The drawing under review shows one solid part. Ordinate dimensions are in mm from its lowest x, y, z. A direction names the side the tool comes from. Give positions to 0.01 mm unless a question says otherwise; leave off trailing zeros. Order: outer loops, then holes, each group sorted by start corner. A loop starts at its lowest first (then second) coordinate and runs counter-clockwise, first axis right, second up. Notation, with made-up numbers: (-7.5, -21.5) - (13.5, -21.5) arc R14 cw to (13.5, 0.5) - close; hole circle Ø8 at (54, -31). An arc over 180 degrees is marked (long way). Answer as a JSON object with one key per item and string values. Group by question number.
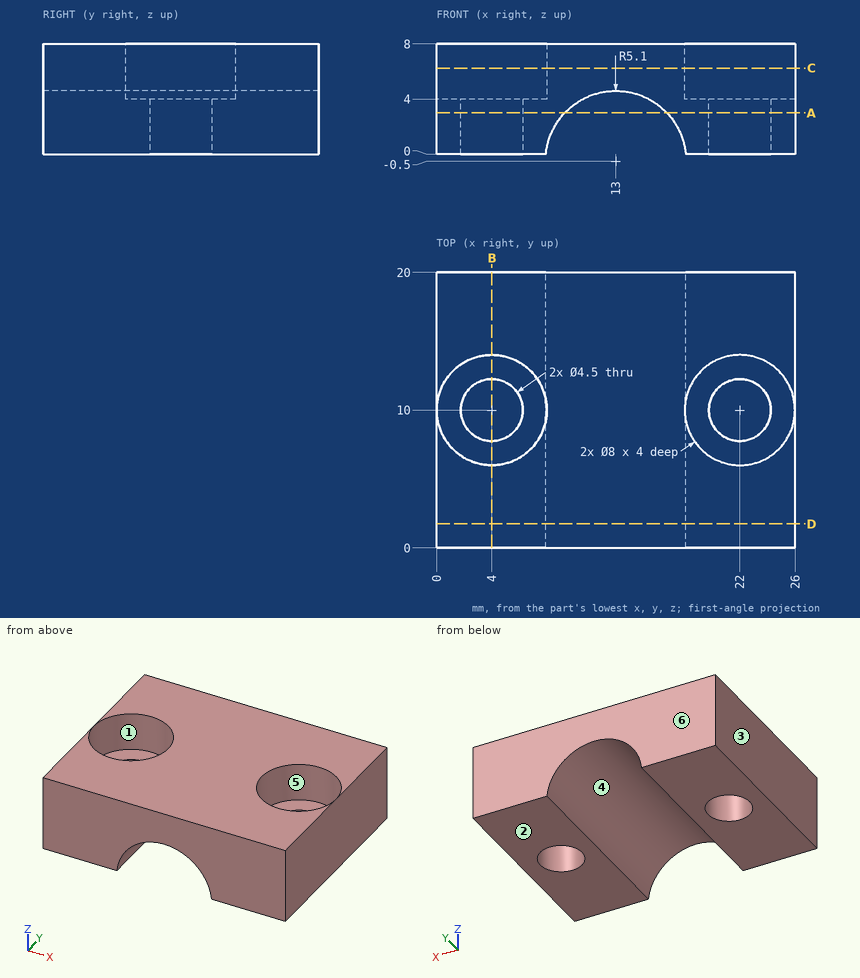
1) For line 1 (Y direction, x = 4, z = 2.1); line 2 (Y direction, x = 22, z = 6.75); line 3 (X direction, y = 10, z = 1.9), list the stretches that pass through material, from the lowest coordinate up.
2) Consider section C-C (z = 6.25). Give the boundary of the cut face in (x, y).
3) Consider section B-B (x = 4). Give the boundary of the cut face in (y, z).
4) Consider section A-A (z = 3). Give the boundary of the cut face in (x, y), plus the area to 3 significant figures.
5) For the marked faces 5 and 6, list the 3-axis set-ups (+Z, -Z, +X, -X, +Y, -Y) from which the entire face can be reached by the end or side of a thin tool; tool diameter is ignored.
6) For pin 1 (2.5 mm diameter, centred on x = 20.5, y = 11, fed in from +Z); pin 2 (9 mm diameter, centred on x = 4, y = 11.5, fed in from +Z); pin 3 (2.5 mm diameter, centred on x = 4, y = 10, fed in from +Z), all flat-tipped, find the tip position at first contact; note any pin that passes through.
7) Consider section D-D (y = 1.75). Give the boundary of the cut face in (x, z), plus the area to 3 significant figures.
8) Mouldability with a two-part tool opening along X and no side actions: class the marked faces 1, 2, 3 and 4 as released by +X, released by -X, zero draft, split by the parting line, or undercut.
Result set:
{
 "1": {"line 1": "y = 0 to 7.75, 12.25 to 20", "line 2": "y = 0 to 6, 14 to 20", "line 3": "x = 0 to 1.75, 6.25 to 8.5, 17.5 to 19.75, 24.25 to 26"},
 "2": {"outline": "(0, 0) - (26, 0) - (26, 20) - (0, 20) - close; hole circle Ø8 at (4, 10); hole circle Ø8 at (22, 10)"},
 "3": {"outline": "(0, 0) - (7.75, 0) - (7.75, 4) - (6, 4) - (6, 8) - (0, 8) - close; (12.25, 0) - (20, 0) - (20, 8) - (14, 8) - (14, 4) - (12.25, 4) - close"},
 "4": {"outline": "(0, 0) - (9.29, 0) - (9.29, 20) - (0, 20) - close; (16.71, 0) - (26, 0) - (26, 20) - (16.71, 20) - close; hole circle Ø4.5 at (4, 10); hole circle Ø4.5 at (22, 10)", "area": "340 mm2"},
 "5": {"face 5": "+Z", "face 6": "+Z, -Z, +X, -X, +Y"},
 "6": {"pin 1": "stops at z = 4", "pin 2": "stops at z = 8", "pin 3": "passes through"},
 "7": {"outline": "(0, 0) - (7.92, 0) arc R5.1 cw to (18.08, 0) - (26, 0) - (26, 8) - (0, 8) - close", "area": "172 mm2"},
 "8": {"face 1": "undercut", "face 2": "zero draft", "face 3": "released by -X", "face 4": "undercut"}
}
